from build123d import *
from OCP.BRepFilletAPI import BRepFilletAPI_MakeChamfer

# Parameters (mm, degrees)
BOSS_EXTRUDE1_DEPTH = 15
CHAMFER1_SIZE       = 20
CHAMFER1_SIZE2      = 24.644345169
CHAMFER2_SIZE       = 20
CHAMFER2_SIZE2      = 24.644345169
CHAMFER3_SIZE       = 20
CHAMFER3_SIZE2      = 24.644345169
CUT_EXTRUDE1_DEPTH  = 411.634172553


with BuildPart() as part:
    # Sketch2 → Boss-Extrude1 (new body)
    with BuildSketch(Plane(origin=(0, 0, 0), x_dir=(1, 0, 0), z_dir=(0, 1, 0))):
        Polygon((-195.090568581, 343.177241046), (-224.999566436, 0), (-184.654847842, 0), (-135.549804353, 279.031716914), (135.549804353, 279.031716914), (184.654847842, 0), (224.999566436, 0), (195.090568581, 343.177241046), align=None)
    extrude(amount=-BOSS_EXTRUDE1_DEPTH)

    # Chamfer1: one chamfer whose edges measure the first distance from different faces: ONE call of the kernel's chamfer builder (chamfer() names one face for all edges)
    chamfer1_edges_1 = [part.edges().sort_by_distance(p)[0] for p in [
        (135.549804353, -7.5, -279.031716914),
    ]]
    chamfer1_side_1 = [part.faces().sort_by_distance(p)[0] for p in [
        (160.102326098, -7.5, -139.515858457),
    ]]
    chamfer1_edges_2 = [part.edges().sort_by_distance(p)[0] for p in [
        (-135.549804353, -7.5, -279.031716914),
    ]]
    chamfer1_side_2 = [part.faces().sort_by_distance(p)[0] for p in [
        (0, -7.5, -279.031716914),
    ]]
    chamfer1 = BRepFilletAPI_MakeChamfer(part.part.solid().wrapped)
    for e in chamfer1_edges_1:
        chamfer1.Add(CHAMFER1_SIZE, CHAMFER1_SIZE2, e.wrapped, chamfer1_side_1[0].wrapped)  # the first distance lies on this face
    for e in chamfer1_edges_2:
        chamfer1.Add(CHAMFER1_SIZE, CHAMFER1_SIZE2, e.wrapped, chamfer1_side_2[0].wrapped)  # the first distance lies on this face
    add(Compound.cast(chamfer1.Shape()), mode=Mode.REPLACE)

    # Chamfer2
    chamfer2_edges = [part.edges().sort_by_distance(p)[0] for p in [
        (184.654847842, -7.5, 0),
    ]]
    chamfer2_side = [part.faces().sort_by_distance(p)[0] for p in [
        (204.827207139, -7.5, 0),
    ]]
    chamfer(chamfer2_edges, length=CHAMFER2_SIZE, length2=CHAMFER2_SIZE2, reference=chamfer2_side[0])

    # Chamfer3
    chamfer3_edges = [part.edges().sort_by_distance(p)[0] for p in [
        (-184.654847842, -7.5, 0),
    ]]
    chamfer3_side = [part.faces().sort_by_distance(p)[0] for p in [
        (-204.827207139, -7.5, 0),
    ]]
    chamfer(chamfer3_edges, length=CHAMFER3_SIZE, length2=CHAMFER3_SIZE2, reference=chamfer3_side[0])

    # Sketch3 → Cut-Extrude1 (cut, through all)
    with BuildSketch(Plane(origin=(0, 0, 0), x_dir=(1, 0, 0), z_dir=(0, 1, 0))):
        Polygon((200.68105686, 279.031716914), (185.737267566, 277.729317721), (190.600969481, 221.922974338), (205.544758775, 223.225373531), align=None)
        Polygon((210.40846069, 167.419030149), (195.464671397, 166.116630955), (200.328373312, 110.310287572), (215.272162606, 111.612686766), align=None)
        Polygon((209.942268873, 0), (224.999566436, 0), (220.135864521, 55.806343383), (205.192075227, 54.503944189), align=None)
    cut_extrude1 = extrude(amount=-CUT_EXTRUDE1_DEPTH, mode=Mode.SUBTRACT)

    # Mirror1: Cut-Extrude1 across plane
    add(cut_extrude1.mirror(Plane(origin=(0, 0, 0), x_dir=(0, 0, 1), z_dir=(1, 0, 0))), mode=Mode.SUBTRACT)


solid = part.part
Read the model definition and answer for the solid it produces. Units are mm, in the model's axes. A direction names the side the tool comes from. Give positions to 0.01 mm unless a question says otherwise; leave off trailing zeros. Write each loop counter-clockwise with the first axis right and the second up, starting at its lowest first coordinate (ties: lowest second). Pieces come first, ordered by that corner, then holes. Notation, with made-up numbers: (37.5, -36.75) - (63.5, -36.75) arc R30 ccw to (63.5, -1.75) - close; hole circle Ø8 at (-27.5, -34). An arc over 180 degrees is marked (long way). Use CSV: the item, a comma, the result in double quotes. Start each with the question number.
(1) Given P1, Ø1, axis at y = -8.5, z = -118, coming from the +X side; P2, Ø4.5, axis at x = -15.5, y = -9, coming from the +Z side; P3, Ø2, axis at y = -3.5, z = -240.5, coming from the -X side, each flat-ended and moving along its own axis, determine where each tip first touches the part or whether it passes through.
(2) Find section C-C (x = -104). Give the vertices of the cut face in (y, z).
(3) Determine the mould class of faces 1 (the flat face through (-203.041, -7.395, -166.777)), 2 (the flat face through (-197.847, -7.395, -311.553)), 3 (the flat face through (-3, -15, -288)) for opening direction Z: +Z half, -Z half, draft (parallel to the pull), parting line (faces both ways), or undercut.
(4) Find section A-A (z = -121.5). Give the vertices of the cut face in (x, y).
(5) Consider line 1 along X through (y, z) = (-3.5, -185.5); line 2 along X through (y, z) = (-9.5, -60.5); line 3 along Z through (x, y) = (87, -8.5). Determine where each line is inside the solid, lowest interval first.
(6) For faces 4 (the flat face through (-4, -7, -279.032)), 5 (the flat face through (212.769, -7.395, -55.164)), 6 (the flat face through (-212.769, -7.395, -55.164)), determine the directions among +Z, -Z, +X, -X, +Y, -Y from which every point of the face is accessible in a straight line to the end or side of a thin tool.
(7) Find section D-D (z = -197.5). Give the vertices of the cut face in (x, y), plus the area to 3 significant figures.
Findings below:
1,P1,"x = 199.7"
1,P2,"z = -279.03"
1,P3,"x = -189.07"
2,outline,"(-15, -343.18) - (0, -343.18) - (0, -279.03) - (-15, -279.03) - close"
3,face 1,"undercut"
3,face 2,"-Z half"
3,face 3,"draft"
4,outline,"(-199.35, -15) - (-163.27, -15) - (-163.27, 0) - (-199.35, 0) - close; (163.27, -15) - (199.35, -15) - (199.35, 0) - (163.27, 0) - close"
5,line 1,"-208.83 to -152.01, 152.01 to 208.83"
5,line 2,"-219.73 to -174.01, 174.01 to 219.73"
5,line 3,"-343.18 to -279.03"
6,face 4,"+Z, +Y, -Y"
6,face 5,"+X, +Y, -Y"
6,face 6,"-X, +Y, -Y"
7,outline,"(-207.79, -15) - (-149.9, -15) - (-149.9, 0) - (-207.79, 0) - close; (149.9, -15) - (207.79, -15) - (207.79, 0) - (149.9, 0) - close"
7,area,"1,740 mm2"
